Source: three-view drawing plus pictorial views. Frame: mm from the lowest corner of the part. A direction names the side the tool comes from. Give positions to 0.01 mm unless a question says otherwise; leave off trailing zeros. Loops run counter-clockwise (first coordinate to the right, second up) from the corner with the lowest first, then second, coordinate; pieces in that order, holes last. Notation, with made-up numbers: M 5.25,1.25 L 45.25,1.25 A18 ccw 45.25,24.25 Z; hole C -27,45 d5. An arc over 180 degrees is marked long. Answer as a JSON object with one key per item and string values. Group by question number.
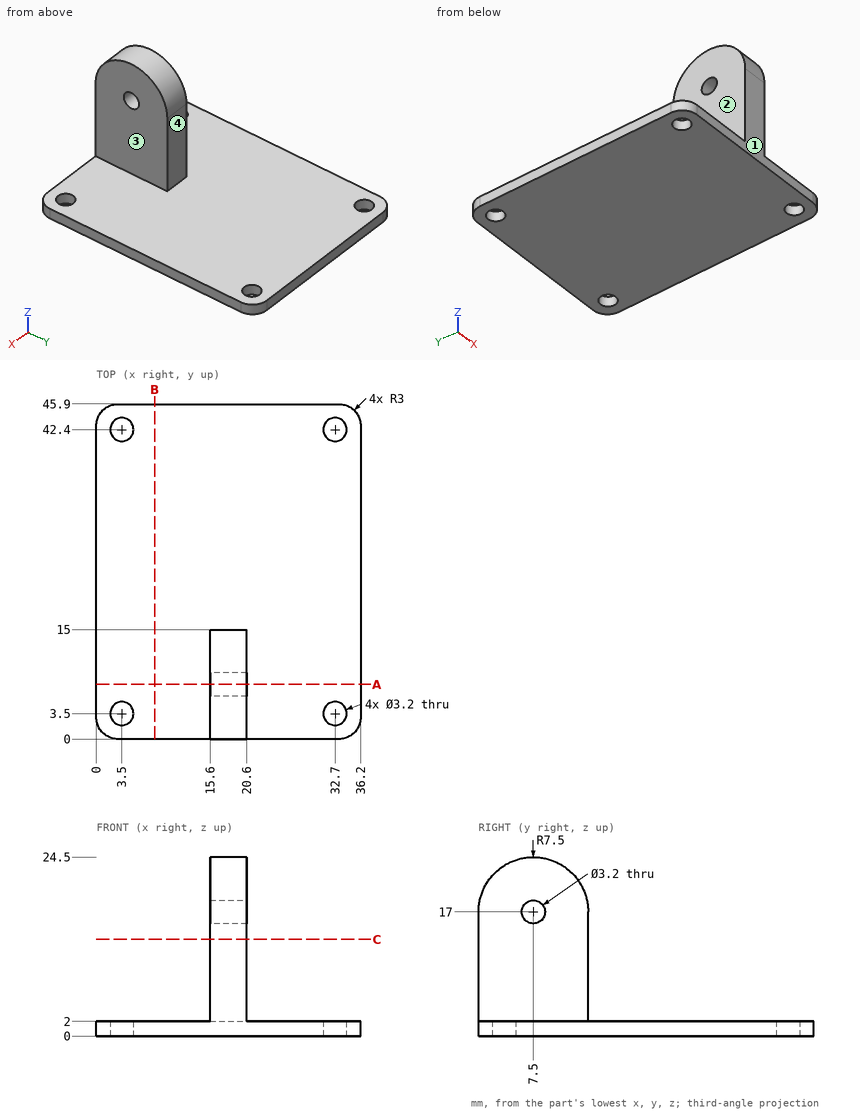
1. Reachability of the marked faces 1, 2, 3 and 4 from +Z, -Z, +X, -X, +Y, -Y: full face, straight path, thin tool, end or side. Return the list, or none.
2. Section C-C (z = 13.25). Output: boundary loops of the cut face in (x, y).
3. Section B-B (x = 8). Output: boundary loops of the cut face in (y, z).
4. Material intervals for L1, parallel to X at y = 3.5, z = 1; L2, parallel to Y at x = 3.5, z = 1.3; L3, parallel to Z at x = 18, y = 7.5, sorted ascending.
5. First-contact query: P1, Ø2.5, axis at x = 18, z = 10, coming from the +Y side; P2, Ø10, axis at y = 14.5, z = 9.5, coming from the +X side; P3, Ø3, axis at x = 22, z = 18.5, coming from the +Y side; P4, Ø12, axis at y = 36.5, z = 2.5, coming from the -X side. Flat tips, straight axial feed; report the tip coordinate or a pass-through.
6. Section A-A (y = 7.5). Output: boundary loops of the cut face in (x, z), then the cut area to 3 significant figures.
Geometry results:
{
 "1": {"face 1": "+Z, -Z, +X, -X, -Y", "face 2": "+Z, -X, +Y, -Y", "face 3": "+Z, +X, +Y, -Y", "face 4": "+Z, +X, -X, +Y"},
 "2": {"outline": "M 15.6,0 L 20.6,0 L 20.6,15 L 15.6,15 Z"},
 "3": {"outline": "M 0,0 L 45.9,0 L 45.9,2 L 0,2 Z"},
 "4": {"L1": "0 to 1.9, 5.1 to 31.1, 34.3 to 36.2", "L2": "0 to 1.9, 5.1 to 40.8, 44 to 45.9", "L3": "0 to 15.4, 18.6 to 24.5"},
 "5": {"P1": "y = 15", "P2": "x = 20.6", "P3": "y = 14.94", "P4": "x = 0"},
 "6": {"outline": "M 0,0 L 36.2,0 L 36.2,2 L 20.6,2 L 20.6,15.4 L 15.6,15.4 L 15.6,2 L 0,2 Z; M 15.6,18.6 L 20.6,18.6 L 20.6,24.5 L 15.6,24.5 Z", "area": "169 mm2"}
}
